Here's the drawing with two shaded views (mm, measured from the low corner). I have some questions. A direction names the side the tool comes from. Coordinates: 2 decimals unless noted, no trailing zeros. Write each loop counter-clockwise with the first axis right and the second up, starting at its lowest first coordinate (ties: lowest second). Pieces come first, ordered by that corner, then holes. Notation, with made-up numbers: (-8, 49) -> (48, 49) arc R7 ccw to (48, 62) -> close; hole circle Ø8 at (-25.75, -6). An arc over 180 degrees is marked (long way). Put each result on its own line as item: value.
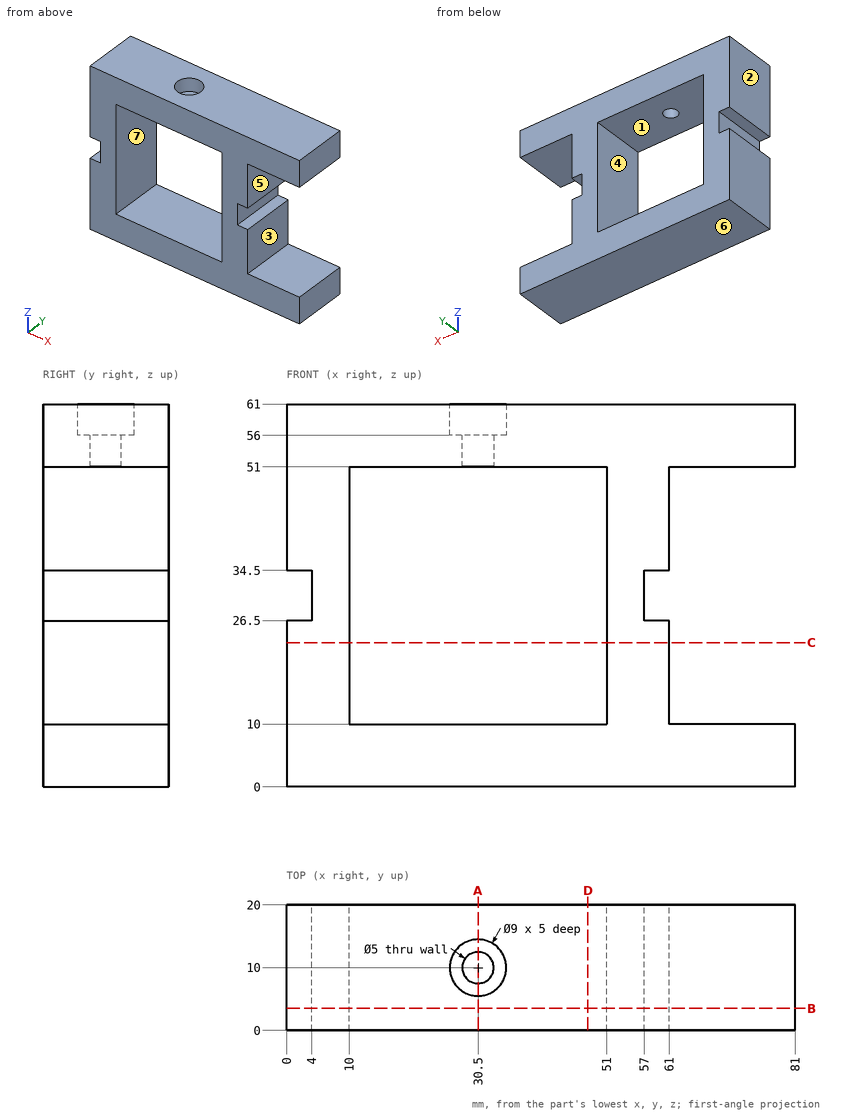
Item 1: Imagine slicing it at C-C on z = 23. Write out the boundary of the cut face in (x, y), then the cut area to 3 significant figures.
Output:
outline: (0, 0) -> (10, 0) -> (10, 20) -> (0, 20) -> close; (51, 0) -> (61, 0) -> (61, 20) -> (51, 20) -> close
area: 400 mm²
Item 2: For P1, Ø8, axis at y = 6, z = 15.5, coming from the +X side; P2, Ø2.5, axis at x = 31, y = 11.5, coming from the +Z side, each with a flat end and sliding along its axis, tell me the tip position at first contact or that it passes through.
Output:
P1: stops at x = 61
P2: stops at z = 56
Item 3: Imagine slicing it at D-D on x = 48. Write out the boundary of the cut face in (y, z).
Output:
outline: (0, 0) -> (20, 0) -> (20, 10) -> (0, 10) -> close; (0, 51) -> (20, 51) -> (20, 61) -> (0, 61) -> close
Item 4: Imagine slicing it at A-A on x = 30.5. Write out the boundary of the cut face in (y, z).
Output:
outline: (0, 0) -> (20, 0) -> (20, 10) -> (0, 10) -> close; (0, 51) -> (7.5, 51) -> (7.5, 56) -> (5.5, 56) -> (5.5, 61) -> (0, 61) -> close; (12.5, 51) -> (20, 51) -> (20, 61) -> (14.5, 61) -> (14.5, 56) -> (12.5, 56) -> close
Item 5: Which directions (+Z, -Z, +X, -X, +Y, -Y) give clear straight access to the entire face, cutting with the end or side of a thin tool? Please do the marked faces 1, 2 and 3.
Output:
face 1: +Y, -Y
face 2: +Z, -Z, -X, +Y, -Y
face 3: +X, +Y, -Y
Item 6: If we mould it in two halves opening along X, with no side actions, what happens to the marked faces 4, 5, 6 and 7? For each: released by +X, released by -X, zero draft, split by the parting line, or undercut.
Output:
face 4: undercut
face 5: released by +X
face 6: zero draft
face 7: undercut
Item 7: Imagine slicing it at B-B on y = 3.5. Write out the boundary of the cut face in (x, z).
Output:
outline: (0, 0) -> (81, 0) -> (81, 10) -> (61, 10) -> (61, 26.5) -> (57, 26.5) -> (57, 34.5) -> (61, 34.5) -> (61, 51) -> (81, 51) -> (81, 61) -> (0, 61) -> (0, 34.5) -> (4, 34.5) -> (4, 26.5) -> (0, 26.5) -> close; hole (10, 10) -> (51, 10) -> (51, 51) -> (10, 51) -> close
Item 8: Please list where these lines run through material, in increasing order: line 1 along Z through (x, y) = (63, 5.75); line 2 along Y through (x, z) = (30.5, 58.8). Write a range as from..to.
Output:
line 1: z = 0..10, 51..61
line 2: y = 0..5.5, 14.5..20
